Source: CAD feature listing. Evaluate the final solid. Frame: model axes, mm. Coordinates: 2 decimals unless noted, no trailing zeros. Order: outer loops, then holes, each group sorted by start corner. A loop starts at its lowest first (then second) coordinate and runs counter-clockwise, first axis right, second up. Notation, with made-up numbers: (-19, 64) -> (35, 64) arc R23 cw to (35, 93) -> close; hole circle Ø9 at (-38.75, 69). An arc over 180 degrees is marked (long way). Put each result on its own line as item: value.
from build123d import *

# Parameters (mm, degrees)
SKETCH1_W           = 7
SKETCH1_H           = 9
BOSS_EXTRUDE1_DEPTH = 19
SKETCH2_R           = 1.984375
CUT_EXTRUDE1_DEPTH  = 9
FILLET1_R           = 3.175


with BuildPart() as part:
    # Sketch1 → Boss-Extrude1 (new body)
    with BuildSketch(Plane.XY):
        with Locations((3.5, 4.5)):
            Rectangle(SKETCH1_W, SKETCH1_H)
    extrude(amount=BOSS_EXTRUDE1_DEPTH)

    # Sketch2 → Cut-Extrude1 (cut)
    with BuildSketch(Plane(origin=(0, 9, 0), x_dir=(1, 0, 0), z_dir=(0, 1, 0))):
        with Locations((4, -4.5)):
            Circle(SKETCH2_R)
        with Locations((4, -14.5)):
            Circle(SKETCH2_R)
    extrude(amount=-CUT_EXTRUDE1_DEPTH, mode=Mode.SUBTRACT)

    # Fillet1
    fillet1_edges = [part.edges().sort_by_distance(p)[0] for p in [
        (7, 4.5, 19),
        (0, 4.5, 19),
        (7, 4.5, 0),
        (0, 4.5, 0),
    ]]
    fillet(fillet1_edges, radius=FILLET1_R)


solid = part.part
1. Cut plane C-C on x = 4.5. Output: boundary loops of the cut face in (y, z), plus the area to 3 significant figures.
Numbers:
outline: (0, 0.07) -> (9, 0.07) -> (9, 2.58) -> (0, 2.58) -> close; (0, 6.42) -> (9, 6.42) -> (9, 12.58) -> (0, 12.58) -> close; (0, 16.42) -> (9, 16.42) -> (9, 18.93) -> (0, 18.93) -> close
area: 101 mm2
2. Pull-direction query (Z, two-part tool) for faces 1 (the cylindrical face through (6.05, 4.56, 18.09)), 2 (the cylindrical face through (2.018, 4.563, 4.413)), 3 (the cylindrical face through (3.57, 4.563, 16.437)), 4 (the flat face through (3, 0, 9)); classes: pulls with the +Z half, pulls with the -Z half, needs draft (parallel to the pull), parting line crosses it, or undercut.
Numbers:
face 1: pulls with the +Z half
face 2: undercut
face 3: undercut
face 4: needs draft
3. Cut plane A-A on z = 14.5. Output: boundary loops of the cut face in (x, y), plus the area to 3 significant figures.
Numbers:
outline: (0, 0) -> (2.02, 0) -> (2.02, 9) -> (0, 9) -> close; (5.98, 0) -> (7, 0) -> (7, 9) -> (5.98, 9) -> close
area: 27.3 mm2
4. Cut plane B-B on y = 0.75. Output: boundary loops of the cut face in (x, z) (3 decimals).
Numbers:
outline: (0, 3.175) arc R3.175 ccw to (3.175, 0) -> (3.825, 0) arc R3.175 ccw to (7, 3.175) -> (7, 15.825) arc R3.175 ccw to (3.825, 19) -> (3.175, 19) arc R3.175 ccw to (0, 15.825) -> close; hole circle Ø3.969 at (4, 4.5); hole circle Ø3.969 at (4, 14.5)
5. First-contact query: pin 1 (1 mm diameter, centred on x = 5.5, y = 5, fed in from +Z); pin 2 (1 mm diameter, centred on x = 1, y = 3, fed in from +Z). Flat tips, straight axial feed; report the tip coordinate or a pass-through.
Numbers:
pin 1: stops at z = 18.77
pin 2: stops at z = 18.52
6. Cut plane D-D on z = 5.75. Output: boundary loops of the cut face in (x, y), plus the area to 3 significant figures.
Numbers:
outline: (0, 0) -> (2.46, 0) -> (2.46, 9) -> (0, 9) -> close; (5.54, 0) -> (7, 0) -> (7, 9) -> (5.54, 9) -> close
area: 35.3 mm2
7. Ray query, line 1 along Z through (x, y) = (4, 2.5); line 2 along Z through (x, y) = (3.25, 2.5); line 3 along X through (y, z) = (3.5, 4.5). Return the intervals inside material, ascending.
Numbers:
line 1: z = 0 to 2.52, 6.48 to 12.52, 16.48 to 19
line 2: z = 0 to 2.66, 6.34 to 12.66, 16.34 to 19
line 3: x = 0 to 2.02, 5.98 to 7
